Work out the finished part from the listing and answer in its coordinate system (mm). A direction names the side the tool comes from. Coordinates: 2 decimals unless noted, no trailing zeros. Write each loop counter-clockwise with the first axis right and the second up, starting at its lowest first coordinate (ties: lowest second). Pieces come first, ordered by that corner, then holes. Notation, with made-up numbers: M 4.25,46 L 15.25,46 A24 ccw 15.25,73 Z; hole C 1.5,-34.75 d8. An arc over 180 degrees is marked long. Answer as CSV lines item,"result". Start each with the question number.
(1) Find the intervals of material crossed by L1, parallel to Z at x = 3, y = -0.5; L2, parallel to Z at x = -24.5, y = -0.75; L3, parallel to X at y = 0.3, z = -24.25, in increasing order. Write a range as [from, to].
(2) For faces 5 (the flat face through (-19, 1.25, 15)), 6 (the flat face through (-12.67, 0, -20)), 7 (the flat face through (24, 6.25, -34)), determine the directions among +Z, -Z, +X, -X, +Y, -Y from which every point of the face is accessible in a straight line to the end or side of a thin tool.
(3) A cutting plane is placed at A-A on z = 24.25. Give the vertices of the cut face in (x, y), then the cut area to 3 significant figures.
(4) A cutting plane is placed at D-D on x = -10.5. Give the vertices of the cut face in (y, z).
(5) The mould has two halves that part along Z. Classify faces 1 (the cylindrical face through (22.504, 0.634, -23.212)), 2 (the flat face through (27.67, 0, 1)), 3 (the flat face through (0, 0, 51.8)), 4 (the flat face through (0, 1.25, -1)): released by +Z, released by -Z, zero draft, split by the parting line, or undercut.
(6) A cutting plane is placed at B-B on y = 3. Count the separate pieces of the cut face and the enclosed holes in it, then the cut area to 3 significant figures.
(7) Flat-ended cylindrical pins translate along their axes: P1, Ø2.5, axis at x = 24.5, z = 24.25, coming from the +Y side; P2, Ø6, axis at x = 24.5, z = 24.25, coming from the +Y side. Find the tip coordinate at first contact, or state that the pin passes through.
(8) A cutting plane is placed at C-C on x = -19.05. Give the vertices of the cut face in (y, z) (3 decimals), then the cut area to 3 significant figures.
from build123d import *

# Parameters (mm, degrees)
BOSS_EXTRU_1_DEPTH      = 1.25
BOSS_EXTRU_1_DEPTH_BACK = 1.25
ESQUISSE1_W             = 55.34
ESQUISSE1_H             = 103.6
ESQUISSE1_R             = 1.0065
ESQUISSE2_R             = 2.25
ENL_V_MAT_EXTRU_1_DEPTH = 1.25
ESQUISSE4_R             = 2.5
BOSS_EXTRU_3_DEPTH      = 5
ESQUISSE7_R             = 1.025
ESQUISSE7_R_2           = 1.0125
ENL_V_MAT_EXTRU_2_DEPTH = 5
ESQUISSE8_W             = 25.34
ESQUISSE8_H             = 73.6
ENL_V_MAT_EXTRU_3_DEPTH = 59.939535967
ESQUISSE16_W            = 25.34
ESQUISSE16_H            = 8
BOSS_EXTRU_6_DEPTH      = 2.5
CONG_8_R                = 1


with BuildPart() as part:
    # Esquisse1 → Boss.-Extru.1 (new, two sides: drawn at the far end of the back side and taken through both)
    with BuildSketch(Plane(origin=(0, 0, 0), x_dir=(1, 0, 0), z_dir=(0, 1, 0)).offset(-BOSS_EXTRU_1_DEPTH_BACK)):
        Rectangle(ESQUISSE1_W, ESQUISSE1_H)
        with Locations(Location((-24.5, -24.25, 0), (0, 0, 270))):
            Circle(ESQUISSE1_R, mode=Mode.SUBTRACT)
        with Locations(Location((-24.5, 24.25, 0), (0, 0, 270))):
            Circle(ESQUISSE1_R, mode=Mode.SUBTRACT)
        with Locations(Location((24.5, 24.25, 0), (0, 0, 270))):
            Circle(ESQUISSE1_R, mode=Mode.SUBTRACT)
        with Locations(Location((24.5, -24.25, 0), (0, 0, 270))):
            Circle(ESQUISSE1_R, mode=Mode.SUBTRACT)
    extrude(amount=BOSS_EXTRU_1_DEPTH + BOSS_EXTRU_1_DEPTH_BACK)

    # Esquisse2 → Enl_v. mat.-Extru.1 (cut)
    with BuildSketch(Plane(origin=(0, 1.25, 0), x_dir=(1, 0, 0), z_dir=(0, 1, 0))):
        with Locations(Location((-24.5, 24.25, 0), (0, 0, 270))):
            Circle(ESQUISSE2_R)
        with Locations(Location((24.5, 24.25, 0), (0, 0, 270))):
            Circle(ESQUISSE2_R)
        with Locations(Location((24.5, -24.25, 0), (0, 0, 270))):
            Circle(ESQUISSE2_R)
        with Locations(Location((-24.5, -24.25, 0), (0, 0, 270))):
            Circle(ESQUISSE2_R)
    extrude(amount=-ENL_V_MAT_EXTRU_1_DEPTH, mode=Mode.SUBTRACT)

    # Esquisse4 → Boss.-Extru.3 (add)
    with BuildSketch(Plane(origin=(0, 1.25, 0), x_dir=(1, 0, 0), z_dir=(0, 1, 0))):
        with Locations(Location((-19.05, -15.24, 0), (0, 0, 270))):
            Circle(ESQUISSE4_R)
        with Locations(Location((-24.13, -45.72, 0), (0, 0, 270))):
            Circle(ESQUISSE4_R)
        with Locations(Location((24.13, -39.37, 0), (0, 0, 270))):
            Circle(ESQUISSE4_R)
        with Locations(Location((24.13, 35.56, 0), (0, 0, 270))):
            Circle(ESQUISSE4_R)
        with Locations(Location((-24.13, 36.83, 0), (0, 0, 270))):
            Circle(ESQUISSE4_R)
    extrude(amount=BOSS_EXTRU_3_DEPTH)

    # Esquisse7 → Enl_v. mat.-Extru.2 (cut)
    with BuildSketch(Plane(origin=(0, 6.25, 0), x_dir=(1, 0, 0), z_dir=(0, 1, 0))):
        with Locations(Location((-24.13, -45.72, 0), (0, 0, 270))):
            Circle(ESQUISSE7_R)
        with Locations(Location((-24.13, 36.83, 0), (0, 0, 270))):
            Circle(ESQUISSE7_R_2)
        with Locations(Location((24.13, -39.37, 0), (0, 0, 270))):
            Circle(ESQUISSE7_R)
        with Locations(Location((24.13, 35.56, 0), (0, 0, 270))):
            Circle(ESQUISSE7_R)
        with Locations(Location((-19.05, -15.24, 0), (0, 0, 270))):
            Circle(ESQUISSE7_R)
    extrude(amount=-ENL_V_MAT_EXTRU_2_DEPTH, mode=Mode.SUBTRACT)

    # Esquisse8 → Enl_v. mat.-Extru.3 (cut, through all)
    with BuildSketch(Plane(origin=(0, 1.25, 0), x_dir=(1, 0, 0), z_dir=(0, 1, 0))):
        Rectangle(ESQUISSE8_W, ESQUISSE8_H)
    extrude(amount=-ENL_V_MAT_EXTRU_3_DEPTH, mode=Mode.SUBTRACT)

    # Esquisse16 → Boss.-Extru.6 (add)
    with BuildSketch(Plane(origin=(0, 1.25, 0), x_dir=(1, 0, 0), z_dir=(0, 1, 0))):
        Rectangle(ESQUISSE16_W, ESQUISSE16_H)
    extrude(amount=-BOSS_EXTRU_6_DEPTH)

    # Cong_8
    cong_8_edges = [part.edges().sort_by_distance(p)[0] for p in [
        (-27.67, 0, -51.8),
        (27.67, 0, -51.8),
        (27.67, 0, 51.8),
        (-27.67, 0, 51.8),
    ]]
    fillet(cong_8_edges, radius=CONG_8_R)


solid = part.part
Here are the results:
1,L1,"z = [-51.8, -36.8], [-4, 4], [36.8, 51.8]"
1,L2,"z = [-51.8, -25.26], [-23.24, 23.24], [25.26, 51.8]"
1,L3,"x = [-27.67, -26.75], [-22.25, -12.67], [12.67, 22.25], [26.75, 27.67]"
2,face 5,"+Y"
2,face 6,"+Y, -Y"
2,face 7,"+Z, -Z, +X, -X, +Y"
3,outline,"M -27.67,-1.25 L -25.51,-1.25 L -25.51,0 L -26.75,0 L -26.75,1.25 L -27.67,1.25 Z; M -23.49,-1.25 L -12.67,-1.25 L -12.67,1.25 L -22.25,1.25 L -22.25,0 L -23.49,0 Z; M 12.67,-1.25 L 23.49,-1.25 L 23.49,0 L 22.25,0 L 22.25,1.25 L 12.67,1.25 Z; M 25.51,-1.25 L 27.67,-1.25 L 27.67,1.25 L 26.75,1.25 L 26.75,0 L 25.51,0 Z"
3,area,"58.7 mm^2"
4,outline,"M -1.25,-51.8 L 1.25,-51.8 L 1.25,-36.8 L -1.25,-36.8 Z; M -1.25,-4 L 1.25,-4 L 1.25,4 L -1.25,4 Z; M -1.25,36.8 L 1.25,36.8 L 1.25,51.8 L -1.25,51.8 Z"
5,face 1,"undercut"
5,face 2,"zero draft"
5,face 3,"released by +Z"
5,face 4,"undercut"
6,separate pieces,"5"
6,enclosed holes,"5"
6,area,"81.8 mm^2"
7,P1,"stops at y = 0"
7,P2,"stops at y = 1.25"
8,outline,"M -1.25,-51.8 L 1.25,-51.8 L 1.25,12.74 L 6.25,12.74 L 6.25,14.215 L 1.25,14.215 L 1.25,16.265 L 6.25,16.265 L 6.25,17.74 L 1.25,17.74 L 1.25,51.8 L -1.25,51.8 Z"
8,area,"274 mm^2"
